Part model, mm, in its own coordinate system. Round coordinates to 2 decimals unless told otherwise and drop trailing zeros. Write each loop counter-clockwise with the first axis right and the second up, starting at its lowest first coordinate (ties: lowest second). Pieces come first, ordered by that corner, then holes.
1) Drill centre lines: L1, parallel to Y at x = 189, z = 0.75; L2, parallel to X at y = 135, z = 1.2; L3, parallel to X at y = 133, z = 2.65. Where is each one in solid material? Low to high.
2) Saw through at C-C on z = 1.85. Write the cut outline in (x, y), and give its area (3 significant figures).
3) Saw through at D-D on y = 150. Write the cut outline in (x, z).
4) Flat gauge pins, fed straight in: pin 1 (0.9 mm diameter, centred on x = 21, z = 2, fed in from -Y); pin 2 (0.9 mm diameter, centred on y = 4.5, z = 1, fed in from +X); pin 3 (1.5 mm diameter, centred on x = 258.5, z = 1.5, fed in from +Y). Where does each tip first touch, or does it go through?
5) Saw through at B-B on x = 195. Write the cut outline in (y, z).
6) Saw through at A-A on y = 113.5. Write the cut outline in (x, z), and give its area (3 significant figures).
```python
from build123d import *

# Parameters (mm, degrees)
BOSS_EXTRU_1_DEPTH      = 3
ENL_V_MAT_EXTRU_1_DEPTH = 345.268848431
ESQUISSE4_W             = 10
ESQUISSE4_H             = 10
ENL_V_MAT_EXTRU_2_DEPTH = 331.898715622
ENL_V_START             = -3
ENL_V_MAT_EXTRU_3_DEPTH = 3
CONG_2_R                = 10
ENL_V_MAT_EXTRU_4_DEPTH = 331.274729043


# Read off the part's stored shape, not the designer's step: Enl_v. mat.-Extru.3
with BuildPart() as part:
    # Esquisse1 → Boss.-Extru.1 (new body)
    with BuildSketch(Plane.XY):
        Polygon((0, 0), (0, 127.45), (65.1, 200), (215.1, 200), (280.2, 127.45), (280.2, 0), align=None)
    extrude(amount=BOSS_EXTRU_1_DEPTH)

    # Esquisse2 → Enl_v. mat.-Extru.1 (cut, through all)
    with BuildSketch(Plane(origin=(0, 0, 0), x_dir=(-1, 0, 0), z_dir=(0, 0, -1))):
        Polygon((-16.6, 0), (-16.6, 145.969439351), (0, 127.45), (0, 0), align=None)
        Polygon((-280.2, 127.45), (-263.6, 145.969439351), (-263.6, 0), (-280.2, 0), align=None)
    extrude(amount=-ENL_V_MAT_EXTRU_1_DEPTH, mode=Mode.SUBTRACT)

    # Esquisse4 → Enl_v. mat.-Extru.2 (cut, through all)
    with BuildSketch(Plane.XY.offset(3)):
        with Locations((21.6, 5)):
            Rectangle(ESQUISSE4_W, ESQUISSE4_H)
        with Locations((21.6, 57.4)):
            Rectangle(ESQUISSE4_W, ESQUISSE4_H)
        with Locations((258.6, 131)):
            Rectangle(ESQUISSE4_W, ESQUISSE4_H)
        with Locations((21.6, 131)):
            Rectangle(ESQUISSE4_W, ESQUISSE4_H)
        with Locations((258.6, 57.4)):
            Rectangle(ESQUISSE4_W, ESQUISSE4_H)
        with Locations((258.6, 5)):
            Rectangle(ESQUISSE4_W, ESQUISSE4_H)
    extrude(amount=-ENL_V_MAT_EXTRU_2_DEPTH, mode=Mode.SUBTRACT)

    # Enl_v. mat.-Extru.3 outline → Enl_v. mat.-Extru.3 (cut)
    with BuildSketch(Plane.XY.offset(3).offset(ENL_V_START)):
        with BuildLine():
            ThreePointArc((64.94882545, 199.831525137), (89.550086935, 185.958261713), (95.898092872, 158.4375))
            ThreePointArc((95.898092872, 158.4375), (140.1, 105), (184.301907128, 158.4375))
            ThreePointArc((184.301907128, 158.4375), (190.649913065, 185.958261713), (215.25117455, 199.831525137))
            Line((215.25117455, 199.831525137), (215.1, 200))
            Line((215.1, 200), (65.1, 200))
            Line((65.1, 200), (64.94882545, 199.831525137))
        make_face()
    extrude(amount=ENL_V_MAT_EXTRU_3_DEPTH, mode=Mode.SUBTRACT)

    # Cong_2
    cong_2_edges = [part.edges().sort_by_distance(p)[0] for p in [
        (64.94882545, 199.831525137, 1.5),
        (215.25117455, 199.831525137, 1.5),
    ]]
    fillet(cong_2_edges, radius=CONG_2_R)

    # Esquisse6 → Enl_v. mat.-Extru.4 (cut, through all)
    with BuildSketch(Plane.XY.offset(3)):
        Polygon((253.6, 136), (162.037145506, 136), (157.83002171, 194.744262237), (193.590573974, 207.065124781), (241.070971096, 207.065124781), (283.142209053, 167.698466408), (280.738138313, 136), (273.47498576, 135.479830357), align=None)
    extrude(amount=-ENL_V_MAT_EXTRU_4_DEPTH, mode=Mode.SUBTRACT)


solid = part.part
```
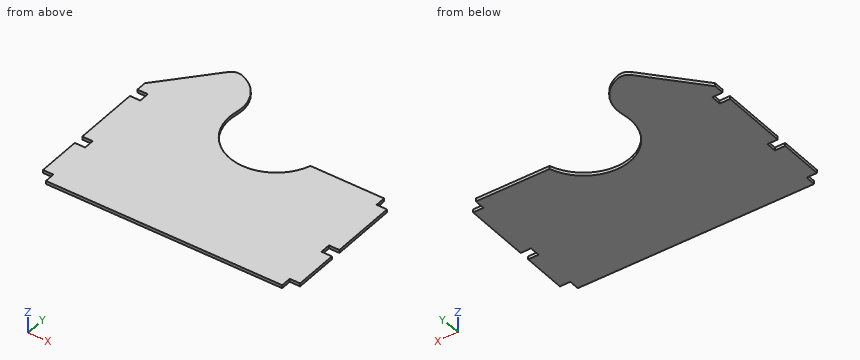
Completed:
1. L1: y = 0 to 136
1. L2: x = 26.6 to 97.67, 182.53 to 253.6
1. L3: x = 26.6 to 98.43, 181.77 to 253.6
2. outline: (16.6, 10) - (26.6, 10) - (26.6, 0) - (253.6, 0) - (253.6, 10) - (263.6, 10) - (263.6, 52.4) - (253.6, 52.4) - (253.6, 62.4) - (263.6, 62.4) - (263.6, 126) - (253.6, 126) - (253.6, 136) - (182.87, 136) arc R45 cw to (95.9, 158.44) arc R35 ccw to (71.48, 198.55) arc R10 ccw to (61.19, 195.64) - (16.6, 145.95) - (16.6, 136) - (26.6, 136) - (26.6, 126) - (16.6, 126) - (16.6, 62.4) - (26.6, 62.4) - (26.6, 52.4) - (16.6, 52.4) - close
2. area: 34,600 mm2
3. outline: (20.23, 0) - (95.1, 0) - (95.1, 3) - (20.23, 3) - close
4. pin 1: stops at y = 10
4. pin 2: stops at x = 253.6
4. pin 3: stops at y = 126
5. outline: (0, 0) - (136, 0) - (136, 3) - (0, 3) - close
6. outline: (16.6, 0) - (113.78, 0) - (113.78, 3) - (16.6, 3) - close; (166.42, 0) - (263.6, 0) - (263.6, 3) - (166.42, 3) - close
6. area: 583 mm2
